Autodesk Inventor part; units mm, degrees
ref_plane "YZ Plane" through (0, 0, 0) normal (1, 0, 0) x (0, 1, 0)
ref_plane "XZ Plane" through (0, 0, 0) normal (0, 1, 0) x (-1, 0, 0)
ref_plane "XY Plane" through (0, 0, 0) normal (0, 0, 1) x (1, 0, 0)
sketch "Sketch1" plane through (0, 0, 0) normal (0, 1, 0) x (-1, 0, 0)
  line L0 (66.7958, 75.9213) -> (-52.5842, 75.9213)
  line L1 (-52.5842, 75.9213) -> (-52.5842, -44.2207)
  line L2 (-52.5842, -44.2207) -> (66.7958, -44.2207)
  line L3 (66.7958, -44.2207) -> (66.7958, 75.9213)
  line L4 (76.9558, 86.0813) -> (-62.7442, 86.0813)
  line L5 (-62.7442, 86.0813) -> (-62.7442, -54.3807)
  line L6 (-62.7442, -54.3807) -> (76.9558, -54.3807)
  line L7 (76.9558, -54.3807) -> (76.9558, 86.0813)
  point P0 (0, 0)
  dimension "d0" = 119.38
  dimension "d1" = 120.142
  dimension "d2" = 10.16
  dimension "d3" = 10.16
  dimension "d4" = 10.16
  dimension "d5" = 10.16
extrude "Extrusion1" add sketch "Sketch1" along normal blind 101.6
sketch "Sketch2" plane through (0, 0, 0) normal (0, -1, 0) x (1, 0, 0)
  line L0 (-76.9558, 86.0813) -> (62.7442, 86.0813)
  line L1 (-76.9558, -54.3807) -> (-76.9558, 86.0813)
  line L2 (62.7442, 86.0813) -> (-76.9558, 86.0813)
  line L3 (-76.9558, 86.0813) -> (-76.9558, -54.3807)
  line L4 (-76.9558, -54.3807) -> (62.7442, -54.3807)
  line L5 (62.7442, -54.3807) -> (62.7442, 86.0813)
  point P0 (0, 0)
extrude "Extrusion2" add sketch "Sketch2" along normal blind 12.7
sketch "Sketch3" plane through (62.7442, 101.6, 86.0813) normal (1, 0, 0) x (0, 0, -1)
  circle A0 centre (69.85, -25.4) radius 3.175
  line L0 (0, 0) -> (140.462, 0)
  line L1 (0, -114.3) -> (0, 0)
  point P0 (86.0813, -101.6)
  dimension "d10" = 6.35
  dimension "d11" = 25.4
  dimension "d12" = 69.85
extrude "Extrusion3" cut sketch "Sketch3" against normal blind 177.8
sketch "Sketch4" plane through (-76.9558, 101.6, 86.0813) normal (0, 0, 1) x (1, 0, 0)
  circle A0 centre (69.85, -44.45) radius 3.175
  line L0 (0, 0) -> (139.7, 0)
  line L1 (0, 0) -> (0, -114.3)
  point P0 (76.9558, -101.6)
  dimension "d15" = 6.35
  dimension "d16" = 44.45
  dimension "d17" = 69.85
extrude "Extrusion4" cut sketch "Sketch4" against normal blind 177.8
properties part number "Box" material "Wood (Cherry)"
For this review, take the finished solid that the model builds, in its own axes (mm). A direction names the side the tool comes from. Round coordinates to 2 decimals unless told otherwise and drop trailing zeros. Order: outer loops, then holes, each group sorted by start corner. A loop starts at its lowest first (then second) coordinate and runs counter-clockwise, first axis right, second up.
Q1. Wall thickness on line 1 (X direction, y = 2, z = -11); line 2 (Z direction, x = -40, y = 20); line 3 (Y direction, x = 41.5, z = 42.5): over which ranges is each line inside the solid? List them lowest first.
Findings below:
line 1: x = -76.96 to -66.8, 52.58 to 62.74
line 2: z = -54.38 to -44.22, 75.92 to 86.08
line 3: y = -12.7 to 0
Q2. We need section C-C, the plane z = -18.5. Give the boundary of the cut face in (x, y), plus the area to 3 significant figures.
Findings below:
outline: (-76.96, -12.7) - (62.74, -12.7) - (62.74, 101.6) - (52.58, 101.6) - (52.58, 0) - (-66.8, 0) - (-66.8, 101.6) - (-76.96, 101.6) - close
area: 3,840 mm2
Q3. We need section B-B, the plane x = 31.5. Give the boundary of the cut face in (y, z), plus the area to 3 significant figures.
Findings below:
outline: (-12.7, -54.38) - (101.6, -54.38) - (101.6, -44.22) - (0, -44.22) - (0, 75.92) - (101.6, 75.92) - (101.6, 86.08) - (-12.7, 86.08) - close
area: 3,850 mm2
Q4. Machinability: for faces 1 (the flat face through (52.584, 50, 17)), 2 (the cylindrical face through (57.735, 78.877, 14.524)), which of the approach directions +Z, -Z, +X, -X, +Y, -Y give a long, thin tool a straight path to every point of the face, cutting with its end or side? Answer none if there is none.
Findings below:
face 1: +Y
face 2: +X, -X
Q5. Insertion check: P1, Ø4, axis at y = 76.2, z = 16.23, coming from the +X side; P2, Ø8, axis at x = 8.5, z = 22, coming from the +Y side. Each pin has a flat end and moves straight along its axis. Give the tip position at first contact, or say it passes through.
Findings below:
P1: passes through
P2: stops at y = 0
Q6. We need section A-A, the plane y = 57.15. Give the boundary of the cut face in (x, z), plus the area to 3 significant figures.
Findings below:
outline: (-76.96, -54.38) - (-10.28, -54.38) - (-10.28, -44.22) - (-66.8, -44.22) - (-66.8, 75.92) - (-10.28, 75.92) - (-10.28, 86.08) - (-76.96, 86.08) - close; (-3.93, -54.38) - (62.74, -54.38) - (62.74, 86.08) - (-3.93, 86.08) - (-3.93, 75.92) - (52.58, 75.92) - (52.58, -44.22) - (-3.93, -44.22) - close
area: 5,150 mm2
Q7. Mouldability with a two-part tool opening along Z and no side actions: class faces 3 (the cylindrical face through (-7.79, 54.05, -49.23)), 4 (the flat face through (-8, 44, 86.081)), 5 (the flat face through (-6, 50, -44.221)) as pulls with the +Z half, pulls with the -Z half, needs draft (parallel to the pull), parting line crosses it, or undercut.
Findings below:
face 3: needs draft
face 4: pulls with the +Z half
face 5: undercut
Q8. We need section D-D, the plane y = 91. Give the boundary of the cut face in (x, z).
Findings below:
outline: (-76.96, -54.38) - (62.74, -54.38) - (62.74, 86.08) - (-76.96, 86.08) - close; hole (-66.8, -44.22) - (52.58, -44.22) - (52.58, 75.92) - (-66.8, 75.92) - close
